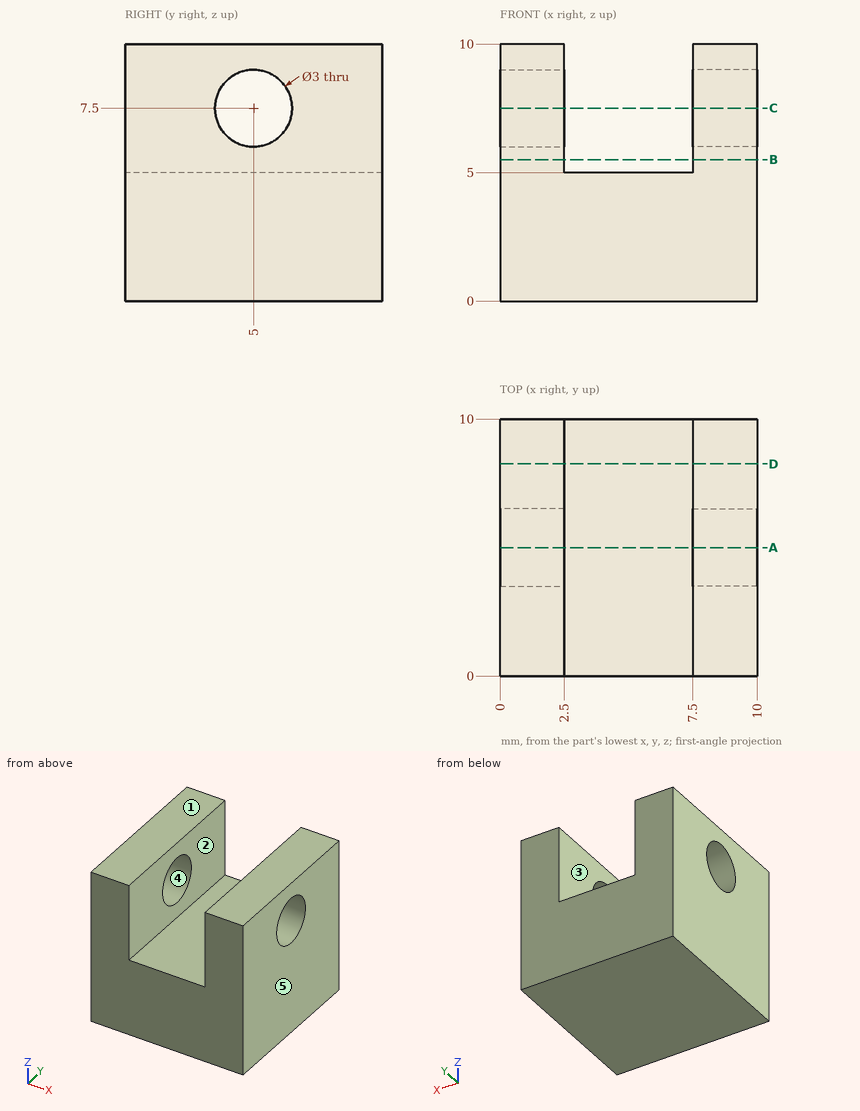
Here's the drawing with two shaded views (mm, measured from the low corner). I have some questions. A direction names the side the tool comes from. Coordinates: 2 decimals unless noted, no trailing zeros. Write each loop counter-clockwise with the first axis right and the second up, starting at its lowest first coordinate (ties: lowest second). Pieces come first, ordered by that corner, then holes. Notation, with made-up numbers: M 68,-34.5 L 103,-34.5 A27 ccw 103,-9.5 Z; hole C -10.75,39.25 d7. An arc over 180 degrees is marked long. Write item = value, one per line. Start each with the question number.
Q1. On a 3-axis mill with a long thin cutter (end or side, diameter ignored), from which of +Z, -Z, +X, -X, +Y, -Y can I reach the whole of each face in a straight line? I mean the marked faces 1 and 2. Say none if no direction works.
Q2. Thinking about a two-plate mould opening in X: for the marked faces 3, 4 and 5, which applies, released by +X, released by -X, zero draft, split by the parting line, or undercut?
Q3. If we section it at C-C, the plane z = 7.5: Write out the boundary of the cut face in (x, y), then the cut area to 3 significant figures.
Q4. I'm going to push a flat-ended pin straight in: pin 1 (4 mm diameter, centred on x = 6.5, z = 6, fed in from +Y). Where does the tip first touch, or does it pass through?
Q5. If I drill on L1, parallel to Z at x = 9.1, y = 5; L2, parallel to Y at x = 9.3, z = 7.5; L3, parallel to X at y = 0.5, z = 7.5, over which ranges is the centre line in solid material (lowest first)? Write a range as [from, to].
Q6. If we section it at B-B, the plane z = 5.5: Write out the boundary of the cut face in (x, y).
Q7. If we section it at D-D, the plane y = 8.25: Write out the boundary of the cut face in (x, z), then the cut area to 3 significant figures.
Q8. If we section it at A-A, the plane y = 5: Write out the boundary of the cut face in (x, z), then the cut area to 3 significant figures.
Check sheet entries:
q1.face_1 = +Z, +X, -X, +Y, -Y
q1.face_2 = +Z, +Y, -Y
q2.face_3 = undercut
q2.face_4 = zero draft
q2.face_5 = released by +X
q3.outline = M 0,0 L 2.5,0 L 2.5,3.5 L 0,3.5 Z; M 0,6.5 L 2.5,6.5 L 2.5,10 L 0,10 Z; M 7.5,0 L 10,0 L 10,3.5 L 7.5,3.5 Z; M 7.5,6.5 L 10,6.5 L 10,10 L 7.5,10 Z
q3.area = 35.0 mm²
q4.pin_1 = 10
q5.L1 = [0, 6], [9, 10]
q5.L2 = [0, 3.5], [6.5, 10]
q5.L3 = [0, 2.5], [7.5, 10]
q6.outline = M 0,0 L 2.5,0 L 2.5,10 L 0,10 Z; M 7.5,0 L 10,0 L 10,10 L 7.5,10 Z
q7.outline = M 0,0 L 10,0 L 10,10 L 7.5,10 L 7.5,5 L 2.5,5 L 2.5,10 L 0,10 Z
q7.area = 75.0 mm²
q8.outline = M 0,0 L 10,0 L 10,6 L 7.5,6 L 7.5,5 L 2.5,5 L 2.5,6 L 0,6 Z; M 0,9 L 2.5,9 L 2.5,10 L 0,10 Z; M 7.5,9 L 10,9 L 10,10 L 7.5,10 Z
q8.area = 60.0 mm²
